```python
from build123d import *

# Parameters (mm, degrees)
SKETCH_W        = 153.5
SKETCH_H        = 59.5
PAD_DEPTH       = 1
SKETCH001_W     = 153.5
SKETCH001_H     = 59.5
SKETCH001_W_2   = 150.5
SKETCH001_H_2   = 56.5
PAD001_DEPTH    = 35
SKETCH002_W     = 6
SKETCH002_H     = 6
PAD002_DEPTH    = 32
SKETCH003_R     = 1
POCKET_DEPTH    = 20
SKETCH004_W     = 4
SKETCH004_H     = 10
SKETCH004_W_2   = 8.1
SKETCH004_H_2   = 8.1
PAD003_DEPTH    = 5
SKETCH005_R     = 1
POCKET001_DEPTH = 5
SKETCH006_W     = 10
SKETCH006_H     = 5
POCKET002_DEPTH = 1.5
FILLET_R        = 1
POCKET003_DEPTH = 4


with BuildPart() as part:
    # Sketch → Pad (new body)
    with BuildSketch(Plane.XY):
        with Locations((76.75, 29.75)):
            Rectangle(SKETCH_W, SKETCH_H)
    extrude(amount=PAD_DEPTH)

    # Sketch001 (on Face6 of Pad) → Pad001 (join)
    with BuildSketch(Plane.XY.offset(1)):
        with Locations((76.75, 29.75)):
            Rectangle(SKETCH001_W, SKETCH001_H)
        with Locations((76.75, 29.75)):
            Rectangle(SKETCH001_W_2, SKETCH001_H_2, mode=Mode.SUBTRACT)
    extrude(amount=PAD001_DEPTH)

    # Sketch002 (on Face15 of Pad001) → Pad002 (join)
    with BuildSketch(Plane.XY.offset(1)):
        with Locations((4.5, 55)):
            Rectangle(SKETCH002_W, SKETCH002_H)
        with Locations((149, 55)):
            Rectangle(SKETCH002_W, SKETCH002_H)
        with Locations((149, 4.5)):
            Rectangle(SKETCH002_W, SKETCH002_H)
        with Locations((4.5, 4.5)):
            Rectangle(SKETCH002_W, SKETCH002_H)
    extrude(amount=PAD002_DEPTH)

    # Sketch003 (on Face15 of Pad002) → Pocket (cut)
    with BuildSketch(Plane.XY.offset(33)):
        with Locations((4.5, 55)):
            Circle(SKETCH003_R)
        with Locations((4.5, 4.5)):
            Circle(SKETCH003_R)
        with Locations((149, 4.5)):
            Circle(SKETCH003_R)
        with Locations((149, 55)):
            Circle(SKETCH003_R)
    extrude(amount=-POCKET_DEPTH, mode=Mode.SUBTRACT)

    # Sketch004 (on Face17 of Pocket) → Pad003 (join)
    with BuildSketch(Plane.XY.offset(1)):
        with Locations((3.5, 38.8)):
            Rectangle(SKETCH004_W, SKETCH004_H)
        with Locations((3.5, 20.7)):
            Rectangle(SKETCH004_W, SKETCH004_H)
        with Locations((49.55, 29.75)):
            Rectangle(SKETCH004_W_2, SKETCH004_H_2)
    extrude(amount=PAD003_DEPTH)

    # Sketch005 (on Face28 of Pad003) → Pocket001 (cut)
    with BuildSketch(Plane.XY.offset(6)):
        with Locations((3.7, 35.45)):
            Circle(SKETCH005_R)
        with Locations((3.7, 24.05)):
            Circle(SKETCH005_R)
    extrude(amount=-POCKET001_DEPTH, mode=Mode.SUBTRACT)

    # Sketch006 (on Face7 of Pocket001) → Pocket002 (cut)
    with BuildSketch(Plane(origin=(0, 0, 0), x_dir=(0, -1, 0), z_dir=(-1, 0, 0))):
        with Locations((-29.75, 4.5)):
            Rectangle(SKETCH006_W, SKETCH006_H)
    extrude(amount=-POCKET002_DEPTH, mode=Mode.SUBTRACT)

    # Fillet
    fillet_edges = [part.edges().sort_by_distance(p)[0] for p in [
        (153.5, 0, 18.5),
        (153.5, 59.5, 18.5),
        (0, 59.5, 18.5),
        (0, 0, 18.5),
    ]]
    fillet(fillet_edges, radius=FILLET_R)

    # Sketch007 (on Face40 of Fillet) → Pocket003 (cut)
    with BuildSketch(Plane.XY.offset(6)):
        Polygon((3, 33.8), (1.5, 33.8), (1.5, 35.3), align=None)
        Polygon((3, 25.7), (1.5, 24.2), (1.5, 25.7), align=None)
    extrude(amount=-POCKET003_DEPTH, mode=Mode.SUBTRACT)


solid = part.part
```
Geometry: final body of the model. Coordinates: model frame, mm. Round coordinates to 2 decimals unless told otherwise and drop trailing zeros. Order: outer loops, then holes, each group sorted by start corner. A loop starts at its lowest first (then second) coordinate and runs counter-clockwise, first axis right, second up. Notation, with made-up numbers: (8, 87) -> (31, 87) arc R26 ccw to (31, 101) -> close; hole circle Ø2 at (32, 30). An arc over 180 degrees is marked (long way). Use CSV: the item, a comma, the result in double quotes. Start each with the question number.
1) Section C-C (y = 47). Return the cut outline in (x, z).
2) Section A-A (y = 32). Return the cut outline in (x, z).
3) Section D-D (x = 119). Return the cut outline in (y, z).
4) First-contact query: pin 1 Ø1.8 at (x, y) = (149, 55) entering from +Z; pin 2 Ø3 at (x, y) = (148.5, 5) entering from +Z; pin 3 Ø3.5 at (x, y) = (2, 27.5) entering from +Z; pin 4 Ø1.5 at (x, y) = (53, 14.5) entering from +Z. Flat tips, straight axial feed; report the tip coordinate or a pass-through.
5) Draft query along Y for faces 1 (the face through (3, 43.8, 3)), 2 (the face through (76, 1, 36)), 3 (the face through (148, 56, 33)), 4 (the face through (76, 59.5, 18)). Return one class per face: +Y half, -Y half, draft (parallel to the pull), parting line (faces both ways), or undercut.
6) Section B-B (z = 17.5). Return the cut outline in (x, y).
7) Material intervals for line 1 along Y through (x, z) = (149, 29); line 2 along Y through (x, z) = (3.7, 4.05); line 3 along X through (y, z) = (24, 4), sorted ascending. Write a range as from..to.
Returned:
1,outline,"(0, 0) -> (153.5, 0) -> (153.5, 36) -> (152, 36) -> (152, 1) -> (1.5, 1) -> (1.5, 36) -> (0, 36) -> close"
2,outline,"(0, 0) -> (153.5, 0) -> (153.5, 36) -> (152, 36) -> (152, 1) -> (53.6, 1) -> (53.6, 6) -> (45.5, 6) -> (45.5, 1) -> (1.5, 1) -> (1.5, 2) -> (0, 2) -> close; (0, 7) -> (1.5, 7) -> (1.5, 36) -> (0, 36) -> close"
3,outline,"(0, 0) -> (59.5, 0) -> (59.5, 36) -> (58, 36) -> (58, 1) -> (1.5, 1) -> (1.5, 36) -> (0, 36) -> close"
4,pin 1,"stops at z = 13"
4,pin 2,"stops at z = 33"
4,pin 3,"stops at z = 36"
4,pin 4,"stops at z = 1"
5,face 1,"undercut"
5,face 2,"draft"
5,face 3,"undercut"
5,face 4,"+Y half"
6,outline,"(0, 1) arc R1 ccw to (1, 0) -> (152.5, 0) arc R1 ccw to (153.5, 1) -> (153.5, 58.5) arc R1 ccw to (152.5, 59.5) -> (1, 59.5) arc R1 ccw to (0, 58.5) -> close; hole (1.5, 7.5) -> (7.5, 7.5) -> (7.5, 1.5) -> (146, 1.5) -> (146, 7.5) -> (152, 7.5) -> (152, 52) -> (146, 52) -> (146, 58) -> (7.5, 58) -> (7.5, 52) -> (1.5, 52) -> close; hole circle Ø2 at (4.5, 4.5); hole circle Ø2 at (4.5, 55); hole circle Ø2 at (149, 4.5); hole circle Ø2 at (149, 55)"
7,line 1,"y = 0..3.5, 5.5..7.5, 52..54, 56..59.5"
7,line 2,"y = 0..7.5, 15.7..23.05, 25.05..25.7, 33.8..34.45, 36.45..43.8, 52..59.5"
7,line 3,"x = 0..2.7, 4.7..5.5, 152..153.5"
